Geometry: final body of the model. Coordinates: model frame, mm. A direction names the side the tool comes from. Give positions to 0.01 mm unless a question says otherwise; leave off trailing zeros. Order: outer loops, then holes, each group sorted by start corner. A loop starts at its lowest first (then second) coordinate and runs counter-clockwise, first axis right, second up. Notation, with made-up numbers: (23.5, 25.5) - (54.5, 25.5) arc R26 ccw to (54.5, 54.5) - close; hole circle Ø6 at (54.5, -34.5). An arc over 180 degrees is marked (long way). One line per item, written item: value.
Autodesk Inventor part; units mm, degrees
ref_plane "YZ Plane" through (0, 0, 0) normal (1, 0, 0) x (0, 1, 0)
ref_plane "XZ Plane" through (0, 0, 0) normal (0, 1, 0) x (-1, 0, 0)
ref_plane "XY Plane" through (0, 0, 0) normal (0, 0, 1) x (1, 0, 0)
sketch "Sketch1" plane through (0, 0, 0) normal (1, 0, 0) x (0, 1, 0)
  circle A0 centre (0, 0) radius 12.7
  line L0 (24.892, 30.48) -> (-25.908, 30.48)
  line L1 (-25.908, 30.48) -> (-25.908, -25.4)
  line L2 (-25.908, -25.4) -> (24.892, -25.4)
  line L3 (24.892, -25.4) -> (24.892, 30.48)
  dimension "d0" = 25.4
  dimension "d1" = 55.88
  dimension "d4" = 25.4
  dimension "d5" = 24.892
  dimension "d6" = 50.8
extrude "Extrusion1" add sketch "Sketch1" along normal blind 6.35
sketch "Sketch2" plane through (0, -25.908, 30.48) normal (0, 0, 1) x (1, 0, 0)
  line L0 (0, 50.8) -> (0, 0)
  line L1 (0, 0) -> (6.35, 0)
  line L2 (6.35, 50.8) -> (6.35, 0)
  line L3 (0, 50.8) -> (6.35, 50.8)
  point P0 (0, 25.908)
  point P1 (3.175, 46.99)
  point P2 (3.175, 3.81)
  dimension "d9" = 6.35
  dimension "d10" = 3.175
  dimension "d11" = 3.175
  dimension "d12" = 3.81
  dimension "d13" = 3.81
hole "Hole1" at (3.175, 21.082, 30.48) at (3.175, -22.098, 30.48) direction (0, 0, -1) diameter 1.9304 depth 7.6708 tip angle 118
sketch "Sketch3" plane through (6.35, 0, 0) normal (1, 0, 0) x (0, 0, -1)
  point P0 (0, 0)
  point P1 (10.4798, 11.5154)
  point P2 (-4.7327, 14.8335)
  point P3 (-15.2125, 3.3181)
  point P4 (-10.4798, -11.5154)
  point P5 (4.7327, -14.8335)
  point P6 (15.2125, -3.3181)
  dimension "d21" = 15.5702
  dimension "d24" = 360
hole "Hole2" at (6.35, 11.5154, -10.4798) at (6.35, 14.8335, 4.7327) at (6.35, 3.3181, 15.2125) at (6.35, -11.5154, 10.4798) at (6.35, -14.8335, -4.7327) at (6.35, -3.3181, -15.2125) direction (-1, 0, 0) diameter 2.3368 end through all
sketch "Sketch5" plane through (0, -25.908, -25.4) normal (0, -1, 0) x (1, 0, 0)
  line L0 (0, 55.88) -> (0, 0)
  line L1 (0, 0) -> (6.35, 0)
  line L2 (6.35, 55.88) -> (6.35, 0)
  line L3 (0, 55.88) -> (6.35, 55.88)
  point P0 (0, 25.4)
  point P1 (3.175, 6.35)
  point P2 (3.175, 49.53)
  dimension "d42" = 6.35
  dimension "d43" = 6.35
hole "Hole4" at (3.175, -25.908, -19.05) at (3.175, -25.908, 24.13) direction (0, 1, 0) diameter 1.9304 depth 7.6708 tip angle 118
properties part number "motor mount"
1) First-contact query: pin 1 (1.9 mm diameter, centred on y = -14.83, z = -4.73, fed in from +X). Flat tip, straight axial feed; report the tip coordinate or a pass-through.
Answers below:
pin 1: through
2) Section B-B, the plane y = 0. Return loops of the section in (x, z), then the cut area to 3 significant figures.
Answers below:
outline: (0, -25.4) - (6.35, -25.4) - (6.35, -12.7) - (0, -12.7) - close; (0, 12.7) - (6.35, 12.7) - (6.35, 30.48) - (0, 30.48) - close
area: 194 mm^2
3) Mould query, pull axis Y, two halves, no side actions, for faces 1 (the face through (3, 24.892, 2)), 2 (the face through (3.13, 11.96, -11.56)), 3 (the face through (2.36, -24.4, 23.61)), 4 (the face through (3.13, 3.27, 16.38)). Classes: released by +Y, released by -Y, zero draft, split by the parting line, or undercut.
Answers below:
face 1: released by +Y
face 2: undercut
face 3: zero draft
face 4: undercut
4) Set-up query: faces 5 (the face through (3, -1, -25.4)), 6 (the face through (4.031, -22.543, 23.167)), 7 (the face through (3.545, -19.712, 23.238)). Return all of +Z, -Z, +X, -X, +Y, -Y with unobstructed straight access to the full face (end or side cutting, diameter ignored); none if empty.
Answers below:
face 5: -Z, +X, -X, +Y, -Y
face 6: +Z
face 7: -Y
5) Section C-C, the plane x = 5.5. Return loops of the section in (y, z).
Answers below:
outline: (-25.91, -25.4) - (24.89, -25.4) - (24.89, 30.48) - (-25.91, 30.48) - close; hole circle Ø2.34 at (-14.83, -4.73); hole circle Ø25.4 at (0, 0); hole circle Ø2.34 at (-11.52, 10.48); hole circle Ø2.34 at (-3.32, -15.21); hole circle Ø2.34 at (3.32, 15.21); hole circle Ø2.34 at (11.52, -10.48); hole circle Ø2.34 at (14.83, 4.73)
6) Section A-A, the plane z = 0. Return loops of the section in (x, y).
Answers below:
outline: (0, -25.91) - (6.35, -25.91) - (6.35, -12.7) - (0, -12.7) - close; (0, 12.7) - (6.35, 12.7) - (6.35, 24.89) - (0, 24.89) - close
7) Material intervals for line 1 along X through (y, z) = (-21, -19); line 2 along Z through (x, y) = (2.75, 0); line 3 along Y through (x, z) = (4, -0.5), sorted ascending.
Answers below:
line 1: 0 to 2.21, 4.14 to 6.35
line 2: -25.4 to -12.7, 12.7 to 30.48
line 3: -25.91 to -12.69, 12.69 to 24.89
